from build123d import *

# Parameters (mm, degrees)
F0_W     = 266.7
F0_H     = 227.774866
F1_DEPTH = 6.35


with BuildPart() as f1:
    # F0 (on Front) → F1 (new body)
    with BuildSketch(Plane.XZ):
        with Locations((0, 113.887433)):
            Rectangle(F0_W, F0_H)
        Polygon((-16.60667, 111.031537), (19.314354, 75.110512), (14.824226, 70.620384), (-21.096798, 106.541409), align=None, mode=Mode.SUBTRACT)
        Polygon((63.35911, 59.407147), (61.29365, 65.411843), (109.331217, 81.935528), (111.396677, 75.930832), align=None, mode=Mode.SUBTRACT)
        Polygon((-119.879616, 205.324226), (-115.389488, 209.814354), (-79.468463, 173.89333), (-83.958591, 169.403202), align=None, mode=Mode.SUBTRACT)
    extrude(amount=F1_DEPTH)


solid = f1.part
Input: part model. Units: mm. Frame: model coordinates. A direction names the side the tool comes from. Coordinates: 2 decimals unless noted, no trailing zeros. Loops run counter-clockwise (first coordinate to the right, second up) from the corner with the lowest first, then second, coordinate; pieces in that order, holes last.
Q1. Draft query along X for faces 1 (the face through (-133.35, -3, 112)), 2 (the face through (-2.885, -3.131, 88.329)), 3 (the face through (-2, 0, 115)). Return one class per face: +X half, -X half, draft (parallel to the pull), parting line (faces both ways), or undercut.
Q2. Cut plane A-A (y = -3.75). Output: boundary loops of the cut face in (x, z), then the cut area to 3 significant figures.
Q3. Contact query for a flat-ended pin moving along its axis: pin 1 (3 mm diameter, centred on x = 98, z = 111, fed in from +Y). Output: stop coordinate, or through.
Q4. Material intervals for line 1 (Z direction, x = -118, y = -1); line 2 (Z direction, x = 96.5, y = -2.5); line 3 (X direction, y = -0.5, z = 177), sorted ascending.
Q5. Cut plane B-B (x = -93). Output: boundary loops of the cut face in (y, z), then the cut area to 3 significant figures.
Q6. Set-up query: faces 4 (the face through (84.98, -3.13, 73.56)), 5 (the face through (133.35, -3, 112)). Return all of +Z, -Z, +X, -X, +Y, -Y with unobstructed straight access to the full face (end or side cutting, diameter ignored); none if empty.
Working result:
1. face 1: -X half
1. face 2: undercut
1. face 3: draft
2. outline: (-133.35, 0) - (133.35, 0) - (133.35, 227.77) - (-133.35, 227.77) - close; hole (-119.88, 205.32) - (-83.96, 169.4) - (-79.47, 173.89) - (-115.39, 209.81) - close; hole (-21.1, 106.54) - (14.82, 70.62) - (19.31, 75.11) - (-16.61, 111.03) - close; hole (61.29, 65.41) - (63.36, 59.41) - (111.4, 75.93) - (109.33, 81.94) - close
2. area: 59,800 mm2
3. pin 1: stops at y = 0
4. line 1: z = 0 to 203.44, 207.2 to 227.77
4. line 2: z = 0 to 70.81, 77.52 to 227.77
4. line 3: x = -133.35 to -91.56, -82.58 to 133.35
5. outline: (-6.35, 0) - (0, 0) - (0, 178.44) - (-6.35, 178.44) - close; (-6.35, 187.42) - (0, 187.42) - (0, 227.77) - (-6.35, 227.77) - close
5. area: 1,390 mm2
6. face 4: +Y, -Y
6. face 5: +Z, -Z, +X, +Y, -Y
